Work out the finished part from the listing and answer in its coordinate system (mm). A direction names the side the tool comes from. Round coordinates to 2 decimals unless told otherwise and drop trailing zeros. Loops run counter-clockwise (first coordinate to the right, second up) from the corner with the lowest first, then second, coordinate; pieces in that order, holes last.
```python
from build123d import *

# Parameters (mm, degrees)
SKETCH1_R                = 23.5
SKETCH1_R_2              = 15
BOSS_EXTRUDE1_DEPTH      = 10
SKETCH2_R                = 30
SKETCH2_R_2              = 15
BOSS_EXTRUDE2_DEPTH      = 10
CHAMFER1_SIZE            = 3
SKETCH3_R                = 5
BOSS_EXTRUDE3_DEPTH      = 15
SKETCH4_W                = 10
SKETCH4_H                = 5
BOSS_EXTRUDE5_DEPTH      = 30
BOSS_EXTRUDE5_DEPTH_BACK = 3


with BuildPart() as part:
    # Sketch1 → Boss-Extrude1 (new body)
    with BuildSketch(Plane.XY):
        Circle(SKETCH1_R)
        Circle(SKETCH1_R_2, mode=Mode.SUBTRACT)
    extrude(amount=-BOSS_EXTRUDE1_DEPTH)

    # Sketch2 → Boss-Extrude2 (add)
    with BuildSketch(Plane.XY):
        Circle(SKETCH2_R)
        Circle(SKETCH2_R_2, mode=Mode.SUBTRACT)
    extrude(amount=BOSS_EXTRUDE2_DEPTH)

    # Chamfer1
    chamfer1_edges = [part.edges().sort_by_distance(p)[0] for p in [
        (-23.5, 0, 0),
    ]]
    chamfer(chamfer1_edges, length=CHAMFER1_SIZE)

    # Sketch3 → Boss-Extrude3 (add)
    with BuildSketch(Plane.XY.offset(10)):
        with Locations((0, 22.5)):
            Circle(SKETCH3_R)
        with Locations((19.485571585, -11.25)):
            Circle(SKETCH3_R)
        with Locations((-19.485571585, -11.25)):
            Circle(SKETCH3_R)
    extrude(amount=BOSS_EXTRUDE3_DEPTH)

    # Sketch4 → Boss-Extrude5 (add, two sides)
    with BuildSketch(Plane(origin=(0, 30, 0), x_dir=(1, 0, 0), z_dir=(0, 1, 0))) as boss_extrude5_sk:
        with Locations((0, -5)):
            Rectangle(SKETCH4_W, SKETCH4_H)
    extrude(amount=BOSS_EXTRUDE5_DEPTH)
    extrude(boss_extrude5_sk.sketch, amount=-BOSS_EXTRUDE5_DEPTH_BACK)


solid = part.part
```
1. Which of the six approach directions +Z, -Z, +X, -X, +Y, -Y give full straight-line access (tool end or side, diameter ignored) to faces 1 (the face through (5, 45, 5)), 2 (the face through (-20, -11, 25)), 3 (the face through (0, -27, 0)), 4 (the face through (24.255, -9.748, 17.395)), 5 (the face through (-5, 45, 5))?
Answer key:
face 1: +Z, -Z, +X, +Y
face 2: +Z, +X, -X, +Y, -Y
face 3: -Z
face 4: +Z
face 5: +Z, -Z, -X, +Y
2. Consider probe 1 along Y at (x, z) = (0, -5.75); probe 2 along Z at (x, y) = (9, 18); probe 3 along Y at (x, z) = (0, 1.5). Determine where each line is inside the solid, lowest interval first.
Answer key:
probe 1: y = -23.5 to -15, 15 to 23.5
probe 2: z = -10 to 10
probe 3: y = -30 to -15, 15 to 30
3. Find section D-D (z = 14.5). Write down the section's boundary in (x, y).
Answer key:
outline: circle Ø10 at (-19.49, -11.25); circle Ø10 at (0, 22.5); circle Ø10 at (19.49, -11.25)
4. Find section C-C (z = 6). Write down the section's boundary in (x, y), then the cut area to 3 significant figures.
Answer key:
outline: (-5, 29.58) arc R30 ccw (long way) to (5, 29.58) - (5, 60) - (-5, 60) - close; hole circle Ø30 at (0, 0)
area: 2,420 mm2
5. Given pin 1 (4 mm diameter, centred on y = 43.5, z = 5.5, fed in from -X); pin 2 (8 mm diameter, centred on x = -2, y = 41.5, fed in from +Z); pin 3 (1.5 mm diameter, centred on y = 48.5, z = 5, fed in from +X), each flat-ended and moving along its own axis, determine where each tip first touches the part or whether it passes through.
Answer key:
pin 1: stops at x = -5
pin 2: stops at z = 7.5
pin 3: stops at x = 5
6. Find section A-A (x = 0). Write down the section's boundary in (y, z).
Answer key:
outline: (-30, 0) - (-26.5, 0) - (-23.5, -3) - (-23.5, -10) - (-15, -10) - (-15, 10) - (-30, 10) - close; (15, -10) - (23.5, -10) - (23.5, -3) - (26.5, 0) - (30, 0) - (30, 2.5) - (60, 2.5) - (60, 7.5) - (30, 7.5) - (30, 10) - (27.5, 10) - (27.5, 25) - (17.5, 25) - (17.5, 10) - (15, 10) - close
7. Determine the mould class of faces 6 (the face through (-14.985, 0.66, -0.14)), 7 (the face through (-14.716, -9.748, 17.395)), 8 (the face through (-0.3, -15.3, -10)) for opening direction Y: +Y half, -Y half, draft (parallel to the pull), parting line (faces both ways), or undercut.
Answer key:
face 6: undercut
face 7: parting line
face 8: draft
8. Find section B-B (y = 0). Write down the section's boundary in (x, z), then the cut area to 3 significant figures.
Answer key:
outline: (-30, 0) - (-26.5, 0) - (-23.5, -3) - (-23.5, -10) - (-15, -10) - (-15, 10) - (-30, 10) - close; (15, -10) - (23.5, -10) - (23.5, -3) - (26.5, 0) - (30, 0) - (30, 10) - (15, 10) - close
area: 479 mm2
